```python
from build123d import *

# Parameters (mm, degrees)
BOSS_EXTRUDE1_DEPTH = 5
SKETCH2_R           = 2.5
CUT_EXTRUDE1_DEPTH  = 10
SKETCH3_R           = 5
CUT_EXTRUDE2_DEPTH  = 2
FILLET1_R           = 2


with BuildPart() as part:
    # Sketch1 → Boss-Extrude1 (new body)
    with BuildSketch(Plane.XY):
        Polygon((0, 0), (0, 80), (20, 80), (40, 0), align=None)
    extrude(amount=BOSS_EXTRUDE1_DEPTH)

    # Sketch2 → Cut-Extrude1 (cut)
    with BuildSketch(Plane.XY.offset(5)):
        with Locations((10, 70)):
            Circle(SKETCH2_R)
        with Locations((10, 50)):
            Circle(SKETCH2_R)
        with Locations((10, 30)):
            Circle(SKETCH2_R)
        with Locations((10, 10)):
            Circle(SKETCH2_R)
    extrude(amount=-CUT_EXTRUDE1_DEPTH, mode=Mode.SUBTRACT)

    # Sketch3 → Cut-Extrude2 (cut)
    with BuildSketch(Plane.XY.offset(5)):
        with Locations((10, 70)):
            Circle(SKETCH3_R)
        with Locations((10, 50)):
            Circle(SKETCH3_R)
        with Locations((10, 30)):
            Circle(SKETCH3_R)
        with Locations((10, 10)):
            Circle(SKETCH3_R)
    extrude(amount=-CUT_EXTRUDE2_DEPTH, mode=Mode.SUBTRACT)

    # Fillet1
    fillet1_edges = [part.edges().sort_by_distance(p)[0] for p in [
        (0, 0, 2.5),
        (0, 80, 2.5),
        (20, 80, 2.5),
        (40, 0, 2.5),
    ]]
    fillet(fillet1_edges, radius=FILLET1_R)


solid = part.part
```
Input: part model. Units: mm. Frame: model coordinates. A direction names the side the tool comes from. Coordinates: 2 decimals unless noted, no trailing zeros. Loops run counter-clockwise (first coordinate to the right, second up) from the corner with the lowest first, then second, coordinate; pieces in that order, holes last. Notation, with made-up numbers: M 60,59.5 L 112,59.5 A19 cw 112,77.5 Z; hole C 6.25,0 d10. An arc over 180 degrees is marked long. Use a Markdown table: item, result. Add a question column.
1) Pin query (flat end, axial travel): P1, Ø8, axis at x = 9.5, y = 12, coming from the +Z side; P2, Ø1.5, axis at y = 30.5, z = 1.5, coming from the +X side; P3, Ø5, axis at x = 10, y = 48.5, coming from the +Z side. Return the tip coordinate at first contact, or that it passes through.
2) Section C-C, the plane x = 10. Give the number of separate pieces and of enclosed holes in the cut face, plus the area to 3 significant figures.
3) Section A-A, the plane y = 70. Return the cut outline in (x, z), plus the area to 3 significant figures.
4) Line query: L1, parallel to Y at x = 10, z = 1.75; L2, parallel to Y at x = 10, z = 4.1; L3, parallel to X at y = 28.5, z = 0.55 (3 decimals). Output: solid intervals per line, ascending. Write a range as from..to.
5) Section D-D, the plane y = 10. Return the cut outline in (x, z).
6) Set-up query: faces 4 (the flat face through (16, 32, 0)), 5 (the cylindrical face through (13, 54, 4)). Return all of +Z, -Z, +X, -X, +Y, -Y with unobstructed straight access to the full face (end or side cutting, diameter ignored); none if empty.
7) Draft query along Y for faces 1 (the cylindrical face through (0.57, 0.6, 2.54)), 2 (the flat face through (12, 8, 3)), 3 (the flat face through (16, 32, 5)). Return one class per face: +Y half, -Y half, draft (parallel to the pull), parting line (faces both ways), or undercut.
8) Section B-B, the plane z = 3.9. Return the cut outline in (x, y), plus the area to 3 significant figures.
Answer below:
| question | item | result |
|---|---|---|
| 1 | P1 | z = 5 |
| 1 | P2 | x = 32.56 |
| 1 | P3 | z = 3 |
| 2 | separate pieces | 5 |
| 2 | enclosed holes | 0 |
| 2 | area | 260 mm2 |
| 3 | outline | M 0,0 L 7.5,0 L 7.5,3 L 5,3 L 5,5 L 0,5 Z; M 12.5,0 L 22.5,0 L 22.5,5 L 15,5 L 15,3 L 12.5,3 Z |
| 3 | area | 77.5 mm2 |
| 4 | L1 | 0..7.5, 12.5..27.5, 32.5..47.5, 52.5..67.5, 72.5..80 |
| 4 | L2 | 0..5, 15..25, 35..45, 55..65, 75..80 |
| 4 | L3 | 0..8, 12..32.875 |
| 5 | outline | M 0,0 L 7.5,0 L 7.5,3 L 5,3 L 5,5 L 0,5 Z; M 12.5,0 L 37.5,0 L 37.5,5 L 15,5 L 15,3 L 12.5,3 Z |
| 6 | face 4 | -Z, +X, -X, +Y, -Y |
| 6 | face 5 | +Z |
| 7 | face 1 | -Y half |
| 7 | face 2 | undercut |
| 7 | face 3 | draft |
| 8 | outline | M 0,2 A2 ccw 2,0 L 37.44,0 A2 ccw 39.38,2.49 L 20.38,78.49 A2 ccw 18.44,80 L 2,80 A2 ccw 0,78 Z; hole C 10,10 d10; hole C 10,30 d10; hole C 10,50 d10; hole C 10,70 d10 |
| 8 | area | 2,080 mm2 |
